from build123d import *

# Parameters (mm, degrees)
F0_R      = 52.5
F1_DEPTH  = 130
F2_R      = 47.5
F3_DEPTH  = 125
F5_DEPTH  = 125
F6_R      = 2
F7_W      = 2.493188018
F7_H      = 93.4330150485
F8_DEPTH  = 1.5
F9_R      = 1
F10_W     = 45.0817196397
F10_H     = 2.4400168913
F11_DEPTH = 1.5
F12_R     = 0.99999
F13_W     = 44.996257755
F13_H     = 2.44
F14_DEPTH = 1.5
F15_R     = 0.99999


# Not quite as in the source:
# - a fillet or chamfer is up to 0.001 mm smaller than in the source, because OpenCascade refuses the exact size


with BuildPart() as f1:
    # F0 (on Front) → F1 (new body)
    with BuildSketch(Plane.XZ):
        Circle(F0_R)
    extrude(amount=-F1_DEPTH)

    # F2 (on face) → F3 (cut)
    with BuildSketch(Plane.XZ):
        Circle(F2_R)
    extrude(amount=-F3_DEPTH, mode=Mode.SUBTRACT)

    # F4 (on face) → F5 (cut)
    with BuildSketch(Plane.XZ):
        with BuildLine():
            ThreePointArc((20.9507066756, -42.6300116091), (5.1584797983, -47.2190648591), (-11.2520875409, -46.1480284083))
            Line((-11.2520875409, -46.1480284083), (-11.2520875409, -51.280020729))
            ThreePointArc((-11.2520875409, -51.280020729), (5.0973568866, -52.2519564492), (20.9507066756, -48.1385281224))
            Line((20.9507066756, -48.1385281224), (20.9507066756, -42.6300116091))
        make_face()
    extrude(amount=-F5_DEPTH, mode=Mode.SUBTRACT)

    # F6
    f6_edges = [f1.edges().sort_by_distance(p)[0] for p in [
        (-32.905284, 0, 40.90834),
        (-5.15848, 0, 47.219065),
        (-11.252088, 62.5, -46.148028),
        (20.950707, 62.5, -42.630012),
        (-11.252088, 62.5, -51.280021),
        (20.950707, 62.5, -48.138528),
    ]]
    fillet(f6_edges, radius=F6_R)

    # F7 (on face) → F8 (join)
    with BuildSketch(Plane.XZ.offset(-125)):
        Rectangle(F7_W, F7_H)
    extrude(amount=F8_DEPTH)

    # F9
    f9_edges = [f1.edges().sort_by_distance(p)[0] for p in [
        (-1.246594, 123.5, 0),
        (1.246594, 123.5, 0),
        (0, 123.5, 46.716508),
        (0, 123.5, -46.716508),
    ]]
    fillet(f9_edges, radius=F9_R)

    # F10 (on face) → F11 (join)
    with BuildSketch(Plane.XZ.offset(-125)):
        with Locations((-23.7874538288, -0.268576463)):
            Rectangle(F10_W, F10_H)
    extrude(amount=F11_DEPTH)

    # F12 (radius 1 in the source; OpenCascade refuses exactly that, so slightly less here)
    f12_edges = [f1.edges().sort_by_distance(p)[0] for p in [
        (-23.787454, 123.5, -1.488585),
        (-23.787454, 123.5, 0.951432),
        (-46.328314, 123.5, -0.268576),
        (-1.246594, 123.5, -0.268576),
    ]]
    fillet(f12_edges, radius=F12_R)

    # F13 (on face) → F14 (join)
    with BuildSketch(Plane.XZ.offset(-125)):
        with Locations((23.7447228865, -0.311423186)):
            Rectangle(F13_W, F13_H)
    extrude(amount=F14_DEPTH)

    # F15 (radius 1 in the source; OpenCascade refuses exactly that, so slightly less here)
    f15_edges = [f1.edges().sort_by_distance(p)[0] for p in [
        (23.744723, 123.5, 0.908577),
        (23.744723, 123.5, -1.531423),
        (1.246594, 123.5, -0.311423),
        (46.242852, 123.5, -0.311423),
    ]]
    fillet(f15_edges, radius=F15_R)


solid = f1.part
The listing builds one solid part. Answer for the finished solid, in the listing's coordinates (mm). Round coordinates to 2 decimals unless told otherwise and drop trailing zeros. Write each loop counter-clockwise with the first axis right and the second up, starting at its lowest first coordinate (ties: lowest second). Pieces come first, ordered by that corner, then holes. Notation, with made-up numbers: M -25.5,4.25 L 26.5,4.25 A14 cw 26.5,21.25 Z; hole C 84,25.25 d9. An arc over 180 degrees is marked long. Write each question's results on one line, items separated by ' | '. Start each with the question number.
Item 1: A cutting plane is placed at A-A on y = 39. Write down the section's boundary in (x, z), and give its area (3 significant figures).
Item 2: Flat-ended cylindrical pins translate along their axes: pin 1 Ø3 at (y, z) = (43.5, 4) entering from +X; pin 2 Ø4 at (y, z) = (56.5, 2.5) entering from -X; pin 3 Ø10 at (x, y) = (28.5, 68) entering from +Z. Find the tip coordinate at first contact, or state that the pin passes through.
Item 3: Straight lines are drawn through the part: L1, parallel to X at y = 95.5, z = 0; L2, parallel to Y at x = 18, z = 6; L3, parallel to Z at x = -43.5, y = 32. For each, find the intervals that lie inside material, in ascending order. Write a range as [from, to].
Item 4: For a pull along Z with two mould halves and no side action, classify faces 1 (the face through (10, 125, -2)), 2 (the face through (-3.172, 62.639, 47.394)), 3 (the face through (-6.834, 65.104, 52.053)), 4 (the face through (-49, 0, -10)) as pulls with the +Z half, pulls with the -Z half, needs draft (parallel to the pull), parting line crosses it, or undercut.
Check sheet entries:
1) outline: M -13.78,-50.66 A2 ccw -11.25,-48.73 L -11.25,-47.69 A2 ccw -12.72,-45.77 A47.5 cw long 22.02,-42.09 A2 ccw 20.95,-43.86 L 20.95,-44.98 A2 ccw 23.86,-46.77 A52.5 ccw long Z | area: 1,400 mm²
2) pin 1: x = 52.44 | pin 2: x = -52.5 | pin 3: z = 46.95
3) L1: [-52.5, -47.5], [47.5, 52.5] | L2: [125, 130] | L3: [-29.39, -19.08], [19.08, 29.39]
4) face 1: undercut | face 2: undercut | face 3: parting line crosses it | face 4: needs draft
